Here's the drawing with two shaded views (mm, measured from the low corner). I have some questions. Round coordinates to 2 decimals unless told otherwise and drop trailing zeros. Order: outer loops, then holes, each group sorted by start corner. A loop starts at its lowest first (then second) coordinate and runs counter-clockwise, first axis right, second up.
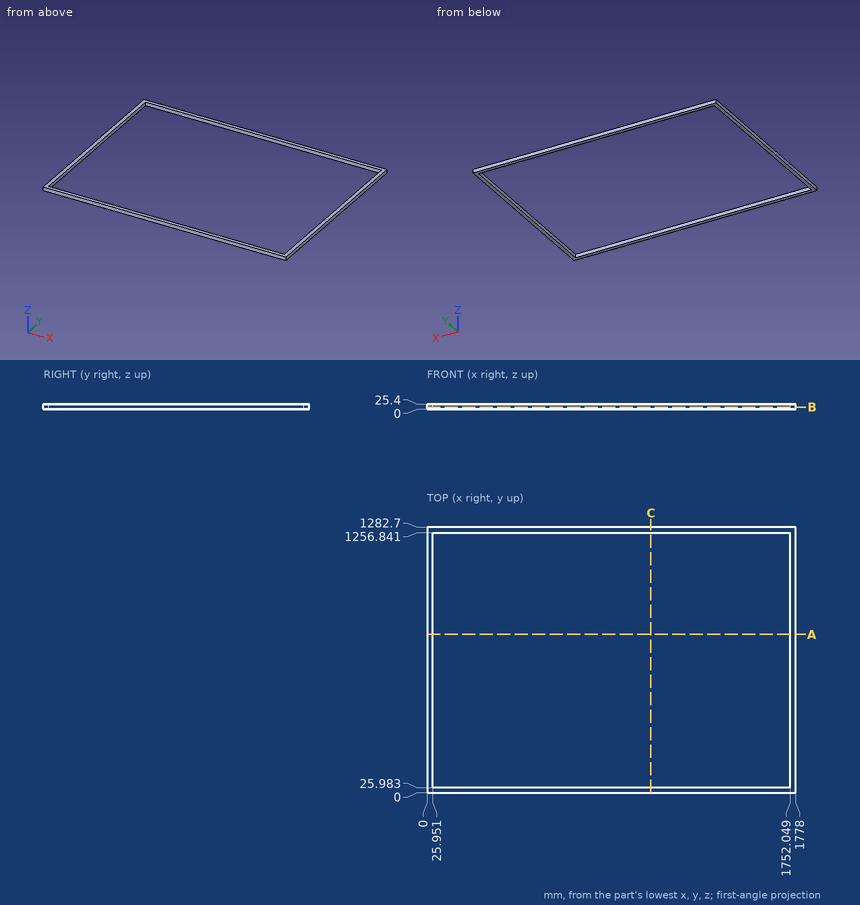
1. If we section it at A-A, the plane y = 765.5: Write out the boundary of the cut face in (x, z), and give its area (3 significant figures).
Evaluation:
outline: (0, 0) - (25.95, 0) - (25.95, 25.4) - (0, 25.4) - close; (1752.05, 0) - (1778, 0) - (1778, 25.4) - (1752.05, 25.4) - close
area: 1,320 mm2
2. If we section it at B-B, the plane z = 9.75: Write out the boundary of the cut face in (x, y), and give its area (3 significant figures).
Evaluation:
outline: (0, 0) - (1778, 0) - (1778, 1282.7) - (0, 1282.7) - close; hole (25.95, 25.98) - (1752.05, 25.98) - (1752.05, 1256.84) - (25.95, 1256.84) - close
area: 156,000 mm2
3. If we section it at C-C, the plane x = 1080: Write out the boundary of the cut face in (y, z).
Evaluation:
outline: (0, 0) - (25.98, 0) - (25.98, 25.4) - (0, 25.4) - close; (1256.84, 0) - (1282.7, 0) - (1282.7, 25.4) - (1256.84, 25.4) - close
4. I need wall thicknesses on probe 1 along Y at (x, z) = (677, 22); probe 2 along X at (y, z) = (433, 24). Which ranges of each line are inside material? Lowest first, please.
Evaluation:
probe 1: y = 0 to 25.98, 1256.84 to 1282.7
probe 2: x = 0 to 25.95, 1752.05 to 1778
